```python
from build123d import *

# Parameters (mm, degrees)
PAD_DEPTH            = 25.25
PAD001_DEPTH         = 37.9
POCKET_DEPTH         = 1.5
SKETCH004_R          = 1.25
SKETCH004_R_2        = 2.5
POCKET001_DEPTH      = 8
POCKET002_DEPTH      = 37.901
POCKET002_DEPTH_BACK = 37.901
SKETCH001_R          = 2.5
POCKET003_DEPTH      = 9


with BuildPart() as part:
    # Sketch → Pad (new body, symmetric)
    with BuildSketch(Plane.XZ):
        Polygon((-21, 30), (-11.5, 30), (-11.5, 29.6), (-4.25, 29.6), (-4.25, 30), (4.25, 30), (4.25, 29.6), (11.5, 29.6), (11.5, 30), (21, 30), (22, 29), (22, 6.1), (20.5, 4.6), (-20.5, 4.6), (-21.6, 5.7), (-21.6, 22), (-22, 22), (-22, 29), align=None)
    extrude(amount=PAD_DEPTH, both=True)

    # Sketch002 → Pad001 (join, symmetric)
    with BuildSketch(Plane.XZ):
        Polygon((-20.6, 29.1), (20.4, 29.1), (21.4, 28.1), (21.4, 5.5), (20.5, 4.6), (-20.5, 4.6), (-21.6, 5.7), (-21.6, 28.1), align=None)
    extrude(amount=PAD001_DEPTH, both=True)

    # Sketch003 (on Face7 of Pad001) → Pocket (cut)
    with BuildSketch(Plane.XZ.offset(37.9)):
        with BuildLine():
            ThreePointArc((-5.25, 24.1), (0, 18.85), (5.25, 24.1))
            Line((5.25, 24.1), (5.25, 29.1))
            Line((-5.25, 29.1), (5.25, 29.1))
            Line((-5.25, 24.1), (-5.25, 29.1))
        make_face()
        with BuildLine():
            ThreePointArc((-19.35, 12.85), (-16.6, 15.6), (-19.35, 18.35))
            Line((-19.35, 18.35), (-21.6, 18.35))
            Line((-21.6, 18.35), (-21.6, 12.85))
            Line((-19.35, 12.85), (-21.6, 12.85))
        make_face()
        with BuildLine():
            ThreePointArc((19.35, 18.35), (16.6, 15.6), (19.35, 12.85))
            Line((19.35, 12.85), (21.4, 12.85))
            Line((21.4, 18.35), (21.4, 12.85))
            Line((19.35, 18.35), (21.4, 18.35))
        make_face()
    pocket = extrude(amount=-POCKET_DEPTH, mode=Mode.SUBTRACT)

    # Sketch004 (on Face42 of Pocket) → Pocket001 (cut)
    with BuildSketch(Plane.XZ.offset(36.4)):
        with Locations((-19.35, 15.6)):
            Circle(SKETCH004_R)
        with Locations((19.35, 15.6)):
            Circle(SKETCH004_R)
        with Locations((0, 24.1)):
            Circle(SKETCH004_R_2)
    pocket001 = extrude(amount=-POCKET001_DEPTH, mode=Mode.SUBTRACT)

    # Mirrored: Pocket001, Pocket across XZ
    add(pocket001.mirror(Plane.XZ), mode=Mode.SUBTRACT)
    add(pocket.mirror(Plane.XZ), mode=Mode.SUBTRACT)

    # Sketch010 → Pocket002 (cut, two sides)
    with BuildSketch(Plane.XZ) as pocket002_sk:
        with BuildLine():
            Line((-9, 0), (-10, 1))
            Line((-10, 1), (-10, 4))
            Line((-10, 4), (-6.6, 7.45))
            Line((-6.6, 7.45), (-6.6, 9.95))
            Line((-6.6, 9.95), (-7.659962205, 11.05))
            ThreePointArc((-7.659962205, 11.05), (-8.2943527546, 12.3411969817), (-9.6, 12.9452882706))
            Line((-9.6, 12.9452882706), (-10, 13.3452882706))
            Line((-10, 13.3452882706), (-10, 14.6952882706))
            Line((-10, 14.6952882706), (-9.6, 15.0952882706))
            ThreePointArc((-9.6, 15.0952882706), (-8.2555446657, 15.738271817), (-7.65, 17.1))
            Line((-7.65, 17.1), (-7.25, 17.5))
            Line((-7.25, 17.5), (0, 17.5))
            Line((0, 17.5), (7.25, 17.5))
            Line((7.25, 17.5), (7.65, 17.1))
            ThreePointArc((7.65, 17.1), (8.2555446657, 15.738271817), (9.6, 15.0952882706))
            Line((9.6, 15.0952882706), (10, 14.6952882706))
            Line((10, 14.6952882706), (10, 13.3452882706))
            Line((10, 13.3452882706), (9.6, 12.9452882706))
            ThreePointArc((9.6, 12.9452882706), (8.2943527546, 12.3411969817), (7.659962205, 11.05))
            Line((7.659962205, 11.05), (6.6, 9.95))
            Line((6.6, 9.95), (6.6, 7.45))
            Line((6.6, 7.45), (10, 4))
            Line((10, 4), (10, 1))
            Line((10, 1), (9, 0))
            Line((4, 0), (9, 0))
            Line((4, 0.4), (4, 0))
            Line((-4, 0.4), (4, 0.4))
            Line((-4, 0), (-4, 0.4))
            Line((-9, 0), (-4, 0))
        make_face()
    extrude(amount=-POCKET002_DEPTH, mode=Mode.SUBTRACT)
    extrude(pocket002_sk.sketch, amount=POCKET002_DEPTH_BACK, mode=Mode.SUBTRACT)

    # Sketch001 (on Face11 of Pad) → Pocket003 (cut)
    with BuildSketch(Plane(origin=(0, 0, 30), x_dir=(-1, 0, 0), z_dir=(0, 0, 1))):
        with Locations((-16, 18)):
            Circle(SKETCH001_R)
        with Locations((-16, -18)):
            Circle(SKETCH001_R)
        with Locations((16, 18)):
            Circle(SKETCH001_R)
        with Locations((16, -18)):
            Circle(SKETCH001_R)
    extrude(amount=-POCKET003_DEPTH, mode=Mode.SUBTRACT)


solid = part.part
```
The listing builds one solid part. Answer for the finished solid, in the listing's coordinates (mm). A direction names the side the tool comes from. Coordinates: 2 decimals unless noted, no trailing zeros. Loops run counter-clockwise (first coordinate to the right, second up) from the corner with the lowest first, then second, coordinate; pieces in that order, holes last. Notation, with made-up numbers: (-4, 44.25) -> (36, 44.25) arc R24 ccw to (36, 79.25) -> close; hole circle Ø11 at (-22, 17.5). An arc over 180 degrees is marked (long way). Return JSON: item names as keys, results as strings. Group by question number.
(1) A cutting plane is placed at B-B on z = 20.25. Write down the section's boundary in (x, y).
(2) Find the intervals of material crossed by probe 1 along X at (y, z) = (-18, 23); probe 2 along Y at (x, z) = (-16, 27.25); probe 3 along X at (y, z) = (32.5, 9), in increasing order. Write a range as from..to.
(3) A cutting plane is placed at A-A on y = -32. Count the separate pieces of the cut face and the enclosed holes in it, and give its area (3 significant figures).
(4) Which of the six approach directions +Z, -Z, +X, -X, +Y, -Y give full straight-line access (tool end or side, diameter ignored) to faces 1 (the flat face through (5.25, -37, 27)), 2 (the cylindrical face through (18.1, 32.46, 15.65)), 3 (the flat face through (20, 37, 12.85)), 4 (the cylindrical face through (-18.16, -32.46, 15.98))?
(5) Determine the mould class of faces 5 (the cylindrical face through (8.2, -0.5, 15.8)), 6 (the cylindrical face through (-16.6, 37.2, 15.5)), 7 (the flat face through (-20, 37, 12.85)) for opening direction X: released by +X, released by -X, zero draft, split by the parting line, or undercut.
(6) A cutting plane is placed at C-C on x = -1.5. Write down the section's boundary in (y, z).
(7) Given pin 1 Ø1.2 at (x, z) = (19.5, 15) entering from -Y; pin 2 Ø5 at (x, y) = (-8, 21) entering from +Z; pin 3 Ø1.5 at (x, z) = (-1, 24.5) entering from +Y, each flat-ended and moving along its own axis, determine where each tip first touches the part or whether it passes through.
The answers:
{
 "1": {"outline": "(-21.6, -37.9) -> (-3.57, -37.9) -> (-3.57, -36.4) -> (3.57, -36.4) -> (3.57, -37.9) -> (21.4, -37.9) -> (21.4, -25.25) -> (22, -25.25) -> (22, 25.25) -> (21.4, 25.25) -> (21.4, 37.9) -> (3.57, 37.9) -> (3.57, 36.4) -> (-3.57, 36.4) -> (-3.57, 37.9) -> (-21.6, 37.9) -> close"},
 "2": {"probe 1": "x = -22..-18.5, -13.5..13.5, 18.5..22", "probe 2": "y = -37.9..-20.5, -15.5..15.5, 20.5..37.9", "probe 3": "x = -21.6..-6.6, 6.6..21.4"},
 "3": {"separate pieces": "1", "enclosed holes": "3", "area": "816 mm^2"},
 "4": {"face 1": "+Z, -Y", "face 2": "+Y", "face 3": "+X, +Y", "face 4": "-Y"},
 "5": {"face 5": "undercut", "face 6": "released by -X", "face 7": "zero draft"},
 "6": {"outline": "(-37.9, 17.5) -> (37.9, 17.5) -> (37.9, 19.07) -> (36.4, 19.07) -> (36.4, 22.1) -> (28.4, 22.1) -> (28.4, 26.1) -> (36.4, 26.1) -> (36.4, 29.1) -> (25.25, 29.1) -> (25.25, 30) -> (-25.25, 30) -> (-25.25, 29.1) -> (-36.4, 29.1) -> (-36.4, 26.1) -> (-28.4, 26.1) -> (-28.4, 22.1) -> (-36.4, 22.1) -> (-36.4, 19.07) -> (-37.9, 19.07) -> close"},
 "7": {"pin 1": "stops at y = -28.4", "pin 2": "stops at z = 29.6", "pin 3": "stops at y = 28.4"}
}
